```python
from build123d import *

# Parameters (mm, degrees)
BOSS_EXTRUDE1_DEPTH = 48.26
SKETCH4_R           = 5.08
BOSS_EXTRUDE2_DEPTH = 38.1
BOSS_EXTRUDE3_START = 25.4
SKETCH5_R           = 5.08
BOSS_EXTRUDE3_DEPTH = 25.4
SKETCH3_W           = 0.9906
SKETCH3_H           = 2.218819971


with BuildPart() as part:
    # Sketch1 → Boss-Extrude1 (new body)
    with BuildSketch(Plane(origin=(0, 0, 0), x_dir=(0, 0, -1), z_dir=(1, 0, 0))):
        Polygon((0, -7.332348419), (6.35, -3.666174209), (6.35, 3.666174209), (0, 7.332348419), (-6.35, 3.666174209), (-6.35, -3.666174209), align=None)
    extrude(amount=BOSS_EXTRUDE1_DEPTH)

    # Sketch4 → Boss-Extrude2 (add)
    with BuildSketch(Plane.ZY):
        with Locations(Location((0, 0, 0), (0, 0, 180))):
            Circle(SKETCH4_R)
    extrude(amount=BOSS_EXTRUDE2_DEPTH)

    # Sketch5 → Boss-Extrude3 (add)
    with BuildSketch(Plane(origin=(48.26, 0, 0), x_dir=(0, 0, -1), z_dir=(1, 0, 0)).offset(BOSS_EXTRUDE3_START)):
        Circle(SKETCH5_R)
    extrude(amount=-BOSS_EXTRUDE3_DEPTH)

    # Sketch3 → Cut-Revolve2 (revolve, cut)
    with BuildSketch(Plane(origin=(0, 0, 0), x_dir=(1, 0, 0), z_dir=(0, 1, 0)), mode=Mode.PRIVATE) as cut_revolve2_sk:
        with Locations((37.0713, 6.824409986)):
            Rectangle(SKETCH3_W, SKETCH3_H)
        with Locations((11.1887, 6.824409986)):
            Rectangle(SKETCH3_W, SKETCH3_H)
    revolve(cut_revolve2_sk.sketch.rotate(Axis((-57.594560376, 0, 0), (1, 0, 0)), 180), axis=Axis((-57.594560376, 0, 0), (1, 0, 0)), mode=Mode.SUBTRACT)


solid = part.part
```
Geometry check sheet. Reference: the model listing, model coordinates, mm. A direction names the side the tool comes from. Coordinates: 2 decimals unless noted, no trailing zeros. Order: outer loops, then holes, each group sorted by start corner. A loop starts at its lowest first (then second) coordinate and runs counter-clockwise, first axis right, second up. Notation, with made-up numbers: M 16,68.5 L 35,68.5 A20 cw 35,107.5 Z; hole C 64.25,-24.5 d3. An arc over 180 degrees is marked long. Answer as a JSON object with one key per item and string values.
Q1. Scan lines: line 1 (X direction, y = -5.25, z = -3); line 2 (Y direction, x = 11.5, z = -0.25); line 3 (X direction, y = 5.5, z = 0.5). Record each from-to range of solid material in increasing order.
Results are:
{"line 1": "x = 0 to 10.69, 11.68 to 36.58, 37.57 to 48.26", "line 2": "y = -5.71 to 5.71", "line 3": "x = 0 to 48.26"}
Q2. Cross-section at C-C on x = 35. Record the cut outline in (y, z), and give its area (3 significant figures).
Results are:
{"outline": "M -7.33,0 L -3.67,-6.35 L 3.67,-6.35 L 7.33,0 L 3.67,6.35 L -3.67,6.35 Z", "area": "140 mm²"}
Q3. Cross-section at A-A on y = 0. Record the cut outline in (x, z) (3 decimals), and give its area (3 significant figures).
Results are:
{"outline": "M -38.1,-5.08 L 0,-5.08 L 0,-6.35 L 10.693,-6.35 L 10.693,-5.715 L 11.684,-5.715 L 11.684,-6.35 L 36.576,-6.35 L 36.576,-5.715 L 37.567,-5.715 L 37.567,-6.35 L 48.26,-6.35 L 48.26,-5.08 L 73.66,-5.08 L 73.66,5.08 L 48.26,5.08 L 48.26,6.35 L 37.567,6.35 L 37.567,5.715 L 36.576,5.715 L 36.576,6.35 L 11.684,6.35 L 11.684,5.715 L 10.693,5.715 L 10.693,6.35 L 0,6.35 L 0,5.08 L -38.1,5.08 Z", "area": "1,260 mm²"}
Q4. Depth check by flat-ended pin: pin 1 Ø6 at (x, z) = (14.5, -2.5) entering from -Y; pin 2 Ø3 at (x, z) = (49, 5) entering from +Y; pin 3 Ø4 at (x, z) = (-8.5, -1.5) entering from -Y. Enter the tip coordinate at first touch or a pass-through.
Results are:
{"pin 1": "stops at y = -7.33", "pin 2": "stops at y = 5.2", "pin 3": "stops at y = -5.08"}
Q5. Release check for a two-part mould opening along X. For faces 1 (the flat face through (43, 0, 6.35)), 2 (the flat face through (48.26, -3.2, 4.3)), 3 (the cylindrical face through (11.196, 3.477, -4.535)) record: released by +X, released by -X, zero draft, split by the parting line, or undercut.
Results are:
{"face 1": "zero draft", "face 2": "released by +X", "face 3": "undercut"}
Q6. Cross-section at B-B on z = -3.25. Record the cut outline in (x, y), and give its area (3 significant figures).
Results are:
{"outline": "M -38.1,-3.9 L 0,-3.9 L 0,-5.46 L 10.69,-5.46 L 10.69,-4.7 L 11.68,-4.7 L 11.68,-5.46 L 36.58,-5.46 L 36.58,-4.7 L 37.57,-4.7 L 37.57,-5.46 L 48.26,-5.46 L 48.26,-3.9 L 73.66,-3.9 L 73.66,3.9 L 48.26,3.9 L 48.26,5.46 L 37.57,5.46 L 37.57,4.7 L 36.58,4.7 L 36.58,5.46 L 11.68,5.46 L 11.68,4.7 L 10.69,4.7 L 10.69,5.46 L 0,5.46 L 0,3.9 L -38.1,3.9 Z", "area": "1,020 mm²"}
Q7. Tool access check on faces 4 (the flat face through (36.576, 6, 0)), 5 (the flat face through (0, -3.2, 4.3)), 6 (the flat face through (23.956, 5.474, -3.219)), 7 (the cylindrical face through (61.138, 5.037, 0.661)). Record the directions out of +Z, -Z, +X, -X, +Y, -Y that give a thin tool (end or side, any length) a straight path to the whole face; none if there is none.
Results are:
{"face 4": "none", "face 5": "-X", "face 6": "-Z, +X, -X, +Y", "face 7": "+X"}
